```python
from build123d import *

# Parameters (mm, degrees)
F0_W      = 95.367364
F0_H      = 68.444572
F0_W_2    = 75.270072
F0_H_2    = 52.89761
F1_DEPTH  = 63.5
F3_DEPTH  = 68.445572
F4_R      = 19.05
F5_DEPTH  = 6.35
F6_R      = 19.05
F7_DEPTH  = 6.35
F8_W      = 76.2
F8_H      = 25.4
F9_DEPTH  = 95.368365
F10_R     = 6.35
F11_DEPTH = 25.4
F12_R     = 6.35
F13_DEPTH = 25.4


with BuildPart() as f1:
    # F0 (on Front) → F1 (new body, symmetric)
    with BuildSketch(Plane.XZ):
        Rectangle(F0_W, F0_H)
        Rectangle(F0_W_2, F0_H_2, mode=Mode.SUBTRACT)
    extrude(amount=F1_DEPTH, both=True)

    # F2 (on face) → F3 (cut, through all)
    with BuildSketch(Plane.XY.offset(34.222286)):
        with BuildLine():
            Line((12.549268, 20.517124), (18.195216, 26.019158))
            ThreePointArc((18.195216, 26.019158), (1.468591, 31.716017), (-15.712911, 27.589254))
            Line((-15.712911, 27.589254), (-11.493717, 21.126547))
            Line((-11.493717, 21.126547), (12.549268, 20.517124))
        make_face()
        with BuildLine():
            Line((-11.493717, 21.126547), (-15.712911, 27.589254))
            ThreePointArc((-15.712911, 27.589254), (-27.295073, 16.218554), (-31.744151, 0.609423))
            Line((-31.744151, 0.609423), (-24.042985, 0.609423))
            Line((-24.042985, 0.609423), (-11.493717, 21.126547))
        make_face()
        with BuildLine():
            ThreePointArc((-17.727481, -26.340063), (-1.43464, -31.717571), (15.277143, -27.832919))
            Line((15.277143, -27.832919), (11.493717, -21.126547))
            Line((11.493717, -21.126547), (-12.549268, -20.517124))
            Line((-12.549268, -20.517124), (-17.727481, -26.340063))
        make_face()
        with BuildLine():
            ThreePointArc((15.277143, -27.832919), (27.166712, -16.432659), (31.744151, -0.609423))
            Line((31.744151, -0.609423), (24.042985, -0.609423))
            Line((24.042985, -0.609423), (11.493717, -21.126547))
            Line((11.493717, -21.126547), (15.277143, -27.832919))
        make_face()
    extrude(amount=-F3_DEPTH, mode=Mode.SUBTRACT)

    # F4 (on face) → F5 (join)
    with BuildSketch(Plane.XY.offset(34.222286)):
        Circle(F4_R)
    extrude(amount=F5_DEPTH)

    # F6 (on face) → F7 (join)
    with BuildSketch(Plane(origin=(0, 0, -34.222286), x_dir=(1, 0, 0), z_dir=(0, 0, -1))):
        Circle(F6_R)
    extrude(amount=F7_DEPTH)

    # F8 (on face) → F9 (cut, through all)
    with BuildSketch(Plane.YZ.offset(47.683682)):
        Rectangle(F8_W, F8_H)
    extrude(amount=-F9_DEPTH, mode=Mode.SUBTRACT)

    # F10 (on face) → F11 (join)
    with BuildSketch(Plane.XY.offset(40.572286)):
        Circle(F10_R)
    extrude(amount=F11_DEPTH)

    # F12 (on face) → F13 (join)
    with BuildSketch(Plane(origin=(0, 0, -40.572286), x_dir=(1, 0, 0), z_dir=(0, 0, -1))):
        Circle(F12_R)
    extrude(amount=F13_DEPTH)


solid = f1.part
```
Input: part model. Units: mm. Frame: model coordinates. A direction names the side the tool comes from. Coordinates: 2 decimals unless noted, no trailing zeros. Write each loop counter-clockwise with the first axis right and the second up, starting at its lowest first coordinate (ties: lowest second). Pieces come first, ordered by that corner, then holes.
1) Pin query (flat end, axial travel): pin 1 Ø3 at (x, y) = (43.5, -15) entering from -Z; pin 2 Ø8 at (x, y) = (17, -25.5) entering from +Z. Return the tip coordinate at first contact, or that it passes through.
2) Section B-B on z = 2. Output: boundary loops of the cut face in (x, y).
3) Material intervals for line 1 along X through (y, z) = (58, -7.5); line 2 along Z through (x, y) = (-1, 42.5); line 3 along Y through (x, z) = (38, 10.5), sorted ascending.
4) Section D-D on z = 38.5. Output: boundary loops of the cut face in (x, y).
5) Section A-A on y = 45. Output: boundary loops of the cut face in (x, z), and give its area (3 significant figures).
6) Set-up query: faces 1 (the flat face through (17.86, -10.72, -30.28)), 2 (the cylindrical face through (-1.38, -6.2, 53.09)), 3 (the flat face through (-1, -1, -26.449)), 4 (the flat face through (-1, 63.5, -30)), 5 (the flat face through (-43, -1, -12.7)). Return all of +Z, -Z, +X, -X, +Y, -Y with unobstructed straight access to the full face (end or side cutting, diameter ignored); none if empty.
7) Section C-C on y = -29.5. Output: boundary loops of the cut face in (x, z), and give its area (3 significant figures).
8) Mould query, pull axis X, two halves, no side actions, for faces 6 (the flat face through (-1, -1, 26.449)), 7 (the flat face through (-43, -1, 12.7)), 8 (the cylindrical face through (-15.12, -11.59, 37.35)). Classes: pulls with the +X half, pulls with the -X half, needs draft (parallel to the pull), parting line crosses it, or undercut.
Check result:
1. pin 1: stops at z = -34.22
1. pin 2: stops at z = 34.22
2. outline: (-47.68, -63.5) - (-37.64, -63.5) - (-37.64, -38.1) - (-47.68, -38.1) - close; (-47.68, 38.1) - (-37.64, 38.1) - (-37.64, 63.5) - (-47.68, 63.5) - close; (37.64, -63.5) - (47.68, -63.5) - (47.68, -38.1) - (37.64, -38.1) - close; (37.64, 38.1) - (47.68, 38.1) - (47.68, 63.5) - (37.64, 63.5) - close
3. line 1: x = -47.68 to -37.64, 37.64 to 47.68
3. line 2: z = -34.22 to -26.45, 26.45 to 34.22
3. line 3: y = -63.5 to -38.1, 38.1 to 63.5
4. outline: circle Ø38.1 at (0, 0)
5. outline: (-47.68, -34.22) - (47.68, -34.22) - (47.68, 34.22) - (-47.68, 34.22) - close; hole (-37.64, -26.45) - (37.64, -26.45) - (37.64, 26.45) - (-37.64, 26.45) - close
5. area: 2,550 mm2
6. face 1: +Z, -Z
6. face 2: +Z
6. face 3: +Y, -Y
6. face 4: +Z, -Z, +X, -X, +Y
6. face 5: +X, -X
7. outline: (-47.68, -34.22) - (-11.74, -34.22) - (-11.74, -26.45) - (-37.64, -26.45) - (-37.64, -12.7) - (-47.68, -12.7) - close; (-47.68, 12.7) - (-37.64, 12.7) - (-37.64, 26.45) - (-11.74, 26.45) - (-11.74, 34.22) - (-47.68, 34.22) - close; (11.74, -34.22) - (47.68, -34.22) - (47.68, -12.7) - (37.64, -12.7) - (37.64, -26.45) - (11.74, -26.45) - close; (11.74, 26.45) - (37.64, 26.45) - (37.64, 12.7) - (47.68, 12.7) - (47.68, 34.22) - (11.74, 34.22) - close
7. area: 1,670 mm2
8. face 6: undercut
8. face 7: needs draft
8. face 8: parting line crosses it
